from build123d import *

# Parameters (mm, degrees)
BOSS_EXTRUDE1_DEPTH     = 10
CUT_EXTRUDE7_START      = -5
CUT_EXTRUDE7_DEPTH      = 5
CUT_EXTRUDE8_DEPTH      = 10.5
CUT_EXTRUDE8_DEPTH_BACK = 10.5
CUT_EXTRUDE9_DEPTH      = 10.5
CUT_EXTRUDE9_DEPTH_BACK = 10.5
SKETCH14_R              = 5
CUT_EXTRUDE10_DEPTH     = 25
BOSS_EXTRUDE2_DEPTH     = 5
CUT_EXTRUDE12_DEPTH     = 5


with BuildPart() as part:
    # Sketch8 → Boss-Extrude1 (new body)
    with BuildSketch(Plane(origin=(0, 0, 0), x_dir=(1, 0, 0), z_dir=(0, 1, 0))):
        with BuildLine():
            Line((15, 0), (305, 0))
            ThreePointArc((305, 0), (315.606601718, 4.393398282), (320, 15))
            Line((320, 15), (320, 85))
            ThreePointArc((320, 85), (315.606601718, 95.606601718), (305, 100))
            Line((305, 100), (15, 100))
            ThreePointArc((15, 100), (4.393398282, 95.606601718), (0, 85))
            Line((0, 85), (0, 15))
            ThreePointArc((0, 15), (4.393398282, 4.393398282), (15, 0))
        make_face()
    extrude(amount=BOSS_EXTRUDE1_DEPTH)

    # Sketch9 → Cut-Extrude7 (cut)
    with BuildSketch(Plane(origin=(0, 10, 0), x_dir=(1, 0, 0), z_dir=(0, 1, 0)).offset(CUT_EXTRUDE7_START)):
        with BuildLine():
            Line((15, 0), (305, 0))
            ThreePointArc((305, 0), (315.606601718, 4.393398282), (320, 15))
            Line((320, 15), (320, 85))
            ThreePointArc((320, 85), (315.606601718, 95.606601718), (305, 100))
            Line((305, 100), (15, 100))
            ThreePointArc((15, 100), (4.393398282, 95.606601718), (0, 85))
            Line((0, 85), (0, 15))
            ThreePointArc((0, 15), (4.393398282, 4.393398282), (15, 0))
        make_face()
        with BuildLine():
            Line((20.5, 94.5), (299.5, 94.5))
            ThreePointArc((299.5, 94.5), (310.106601718, 90.106601718), (314.5, 79.5))
            Line((314.5, 79.5), (314.5, 20.5))
            ThreePointArc((314.5, 20.5), (310.106601718, 9.893398282), (299.5, 5.5))
            Line((299.5, 5.5), (20.5, 5.5))
            ThreePointArc((20.5, 5.5), (9.893398282, 9.893398282), (5.5, 20.5))
            Line((5.5, 20.5), (5.5, 79.5))
            ThreePointArc((5.5, 79.5), (9.893398282, 90.106601718), (20.5, 94.5))
        make_face(mode=Mode.SUBTRACT)
    extrude(amount=CUT_EXTRUDE7_DEPTH, mode=Mode.SUBTRACT)

    # Sketch11 → Cut-Extrude8 (cut, two sides: drawn at the far end of the back side and taken through both)
    with BuildSketch(Plane(origin=(160, 0, 0), x_dir=(0, 0, -1), z_dir=(1, 0, 0)).offset(-CUT_EXTRUDE8_DEPTH_BACK)):
        Polygon((5.5, 10), (5.5, 5), (8, 7.5), align=None)
        Polygon((94.5, 10), (94.5, 5), (92, 7.5), align=None)
    extrude(amount=CUT_EXTRUDE8_DEPTH + CUT_EXTRUDE8_DEPTH_BACK, mode=Mode.SUBTRACT)

    # Sketch13 → Cut-Extrude9 (cut, two sides: drawn at the far end of the back side and taken through both)
    with BuildSketch(Plane.XY.offset(-50).offset(-CUT_EXTRUDE9_DEPTH_BACK)):
        Polygon((314.5, 5), (314.5, 10), (312, 7.5), align=None)
    extrude(amount=CUT_EXTRUDE9_DEPTH + CUT_EXTRUDE9_DEPTH_BACK, mode=Mode.SUBTRACT)

    # Sketch14 → Cut-Extrude10 (cut)
    with BuildSketch(Plane(origin=(0, 0, 0), x_dir=(0, 0, -1), z_dir=(1, 0, 0))):
        with Locations((50, 8)):
            Circle(SKETCH14_R)
    extrude(amount=CUT_EXTRUDE10_DEPTH, mode=Mode.SUBTRACT)

    # Sketch15 → Boss-Extrude2 (add)
    with BuildSketch(Plane(origin=(0, 0, 0), x_dir=(1, 0, 0), z_dir=(0, 1, 0))):
        with BuildLine():
            Line((-7.5, 100), (-7.5, 0))
            Line((-7.5, 0), (15, 0))
            ThreePointArc((15, 0), (4.393398282, 4.393398282), (0, 15))
            Line((0, 15), (0, 85))
            ThreePointArc((0, 85), (4.393398282, 95.606601718), (15, 100))
            Line((15, 100), (-7.5, 100))
        make_face()
    extrude(amount=BOSS_EXTRUDE2_DEPTH)

    # Sketch16 → Cut-Extrude12 (cut)
    with BuildSketch(Plane(origin=(0, 0, 0), x_dir=(1, 0, 0), z_dir=(0, 1, 0))):
        with BuildLine():
            Line((2.5, 0), (-7.5, 0))
            Line((-7.5, 0), (-7.5, 10))
            ThreePointArc((-7.5, 10), (-4.571067812, 2.928932188), (2.5, 0))
        make_face()
        with BuildLine():
            ThreePointArc((-3, 81.648353456), (-6.303408431, 85.25658351), (-7.5, 90))
            Line((-7.5, 90), (-7.5, 10))
            ThreePointArc((-7.5, 10), (-6.303408431, 14.74341649), (-3, 18.351646544))
            Line((-3, 18.351646544), (-3, 50))
            Line((-3, 50), (-3, 81.648353456))
        make_face()
        with BuildLine():
            Line((-7.5, 90), (-7.5, 100))
            Line((-7.5, 100), (2.5, 100))
            ThreePointArc((2.5, 100), (-4.571067812, 97.071067812), (-7.5, 90))
        make_face()
    extrude(amount=CUT_EXTRUDE12_DEPTH, mode=Mode.SUBTRACT)


solid = part.part
Could you check a few things on this model? Use its own coordinates, in mm. A direction names the side the tool comes from. Give positions to 0.01 mm unless a question says otherwise; leave off trailing zeros. Write each loop counter-clockwise with the first axis right and the second up, starting at its lowest first coordinate (ties: lowest second). Pieces come first, ordered by that corner, then holes. Notation, with made-up numbers: (62.5, 62.5) - (67.5, 62.5) arc R29 ccw to (67.5, 95.5) - close; hole circle Ø8 at (12, 69.5). An arc over 180 degrees is marked (long way). Use CSV: the item, a comma, the result in double quotes. Start each with the question number.
Item 1: For faces 4 (the face through (10.01, 7.46, -9.78)), 5 (the face through (9.78, 7.46, -89.99)), 6 (the face through (310.22, 7.46, -10.01)), which set-ups out of +Z, -Z, +X, -X, +Y, -Y let a thin tool reach every point of the face, with its end or its side?
Item 2: I want a section at A-A, the plane z = -50. Please give me the cut outline in (x, y).
Item 3: I want a section at C-C, the plane z = -30. Please give me the cut outline in (x, y).
Item 4: I want a section at B-B, the plane x = 68. Please give me the cut outline in (y, z), then the cut area to 3 significant figures.
Item 5: If we mould it in two halves opening along X, with no side actions, what happens to faces 1 (the face through (154, 0, -51)), 2 (the face through (12, 3, -50)), 3 (the face through (309.99, 7.46, -90.22))? For each: pulls with the +X half, pulls with the -X half, needs draft (parallel to the pull), parting line crosses it, or undercut.
Item 6: If I drill on line 1 along Z through (x, y) = (20.25, 8); line 2 along X through (y, z) = (2.25, -21); line 3 along Z through (x, y) = (222, 8.5), over which ranges is the centre line in solid material (lowest first)?
Item 7: I'm going to push flat-ended pins straight in: pin 1 (3 mm diameter, centred on x = 313.5, y = 7.5, fed in from -Z); pin 2 (1.5 mm diameter, centred on y = 6.5, z = -74, fed in from +X); pin 3 (0.8 mm diameter, centred on y = 8.5, z = -7, fed in from +X). Where does each tip first touch, or does it pass through?
Findings:
1,face 4,"+Z, -X, +Y"
1,face 5,"-Z, -X, +Y"
1,face 6,"+Z, +X, +Y"
2,outline,"(-3, 0) - (320, 0) - (320, 5) - (314.5, 5) - (312, 7.5) - (314.5, 10) - (25, 10) - (25, 3) - (0, 3) - (0, 5) - (-3, 5) - close"
3,outline,"(-3, 0) - (320, 0) - (320, 5) - (314.5, 5) - (314.5, 10) - (5.5, 10) - (5.5, 5) - (-3, 5) - close"
4,outline,"(0, -100) - (5, -100) - (5, -94.5) - (10, -94.5) - (10, -5.5) - (5, -5.5) - (5, 0) - (0, 0) - close"
4,area,"945 mm2"
5,face 1,"needs draft"
5,face 2,"undercut"
5,face 3,"pulls with the +X half"
6,line 1,"z = -94.5 to -55, -45 to -5.5"
6,line 2,"x = -3 to 320"
6,line 3,"z = -94.5 to -5.5"
7,pin 1,"stops at z = -87.79"
7,pin 2,"stops at x = 314.5"
7,pin 3,"stops at x = 306.81"
